Read the model definition and answer for the solid it produces. Units are mm, in the model's axes. Face numbers are marked on the shaded views. Coordinates: 2 decimals unless noted, no trailing zeros. Order: outer loops, then holes, each group sorted by start corner. A loop starts at its lowest first (then second) coordinate and runs counter-clockwise, first axis right, second up.
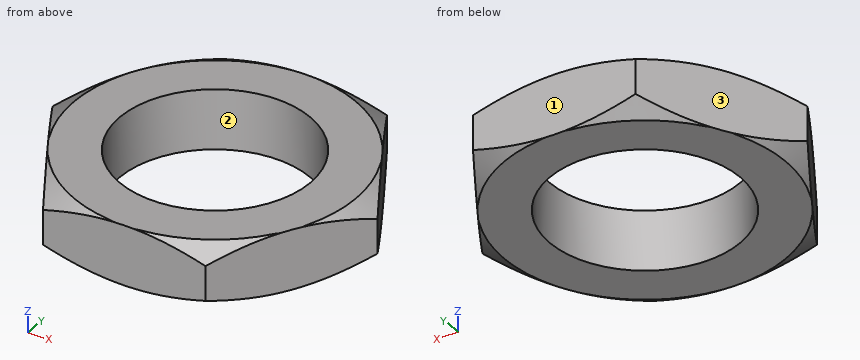
```python
from build123d import *

# Parameters (mm, degrees)
BOSS_EXTRUDE1_DEPTH       = 0.85
SKETCH2_R                 = 15
SKETCH2_R_2               = 4
CUT_EXTRUDE_THIN2_DEPTH   = 1
CUT_EXTRUDE_THIN2_DRAFT   = -60
MIRROR1_COPY_1_SKETCH_R   = 15
MIRROR1_COPY_1_SKETCH_R_2 = 4
MIRROR1_COPY_1_DEPTH      = 1
MIRROR1_COPY_1_DRAFT      = -60
F_1_4_28_TAPPED_HOLE1_D   = 5.4102


with BuildPart() as part:
    # Sketch1 → Boss-Extrude1 (new, symmetric)
    with BuildSketch(Plane.XY):
        Polygon((2.309401077, 4), (-2.309401077, 4), (-4.618802154, 0), (-2.309401077, -4), (2.309401077, -4), (4.618802154, 0), align=None)
    extrude(amount=BOSS_EXTRUDE1_DEPTH, both=True)


with BuildPart() as cut_extrude_thin2_tool:
    # Sketch2 → Cut-Extrude-Thin2 (with draft: the straight prism first)
    with BuildSketch(Plane.XY.offset(0.85)):
        Circle(SKETCH2_R)
        Circle(SKETCH2_R_2, mode=Mode.SUBTRACT)
    extrude(amount=-CUT_EXTRUDE_THIN2_DEPTH)
    # Cut-Extrude-Thin2: the draft: its side faces are tilted about the plane it starts from
    cut_extrude_thin2_sides = [cut_extrude_thin2_tool.faces().sort_by_distance(p)[0] for p in [
        (-15, 0, 0.35),
        (-4, 0, 0.35),
    ]]
    draft(cut_extrude_thin2_sides, Plane.XY.offset(0.85), CUT_EXTRUDE_THIN2_DRAFT)


with BuildPart() as part_1:
    add(part.part)

    # Cut-Extrude-Thin2: cut by cut_extrude_thin2_tool
    add(cut_extrude_thin2_tool.part, mode=Mode.SUBTRACT)


with BuildPart() as mirror1_copy_1_tool:
    # Mirror1 copy 1 sketch → Mirror1 copy 1 (with draft: the straight prism first)
    with BuildSketch(Plane(origin=(0, 0, -0.85), x_dir=(1, 0, 0), z_dir=(0, 0, -1))):
        Circle(MIRROR1_COPY_1_SKETCH_R)
        Circle(MIRROR1_COPY_1_SKETCH_R_2, mode=Mode.SUBTRACT)
    extrude(amount=-MIRROR1_COPY_1_DEPTH)
    # Mirror1 copy 1: the draft: its side faces are tilted about the plane it starts from
    mirror1_copy_1_sides = [mirror1_copy_1_tool.faces().sort_by_distance(p)[0] for p in [
        (-15, 0, -0.35),
        (-4, 0, -0.35),
    ]]
    draft(mirror1_copy_1_sides, Plane(origin=(0, 0, -0.85), x_dir=(1, 0, 0), z_dir=(0, 0, -1)), MIRROR1_COPY_1_DRAFT)


with BuildPart() as part_2:
    add(part_1.part)

    # Mirror1 copy 1: cut by mirror1_copy_1_tool
    add(mirror1_copy_1_tool.part, mode=Mode.SUBTRACT)

    # 1/4-28 Tapped Hole1 (through all)
    with Locations(Plane.XY.offset(0.85)):
        with Locations((0, 0)):
            Hole(F_1_4_28_TAPPED_HOLE1_D / 2)


solid = part_2.part
```
1) A cutting plane is placed at A-A, the plane z = 0.2. Determine the outline of the cut face in (x, y).
A:
outline: (-4.62, 0) - (-2.31, -4) - (2.31, -4) - (4.62, 0) - (2.31, 4) - (-2.31, 4) - close; hole circle Ø5.41 at (0, 0)
2) Determine the mould class of the marked faces 1, 2 and 3 for opening direction X: pulls with the +X half, pulls with the -X half, needs draft (parallel to the pull), parting line crosses it, or undercut.
A:
face 1: needs draft
face 2: undercut
face 3: pulls with the -X half
3) Straight lines are drawn through the part: line 1 (Y direction, x = 2, z = 0.75); line 2 (X direction, y = 1.5, z = 0.55); line 3 (Y direction, x = -0.25, z = -0.1). For each, find the intervals that lie inside material, in ascending order.
A:
line 1: y = -3.66 to -1.82, 1.82 to 3.66
line 2: x = -3.75 to -2.25, 2.25 to 3.75
line 3: y = -4 to -2.69, 2.69 to 4
4) A flat-ended cylindrical pin translates along its axis: pin 1 Ø3 at (x, y) = (0, 0) entering from -Z. Find the tip coordinate at first contact, or state that the pin passes through.
A:
pin 1: passes through
5) A cutting plane is placed at B-B, the plane z = -0.65. Determine the outline of the cut face in (x, y).
A:
outline: (-4.31, -0.53) - (-2.61, -3.47) arc R4.35 ccw to (-1.7, -4) - (1.7, -4) arc R4.35 ccw to (2.61, -3.47) - (4.31, -0.53) arc R4.35 ccw to (4.31, 0.53) - (2.61, 3.47) arc R4.35 ccw to (1.7, 4) - (-1.7, 4) arc R4.35 ccw to (-2.61, 3.47) - (-4.31, 0.53) arc R4.35 ccw to start; hole circle Ø5.41 at (0, 0)
